Could you check a few things on this model? Use its own coordinates, in mm. A direction names the side the tool comes from. Give positions to 0.01 mm unless a question says otherwise; leave off trailing zeros. Write each loop counter-clockwise with the first axis right and the second up, starting at its lowest first coordinate (ties: lowest second). Pieces come first, ordered by that corner, then holes. Notation, with made-up numbers: M 30.5,78 L 66.5,78 A21 ccw 66.5,94 Z; hole C -6.5,-29.75 d2. An arc over 180 degrees is marked long. One line per item, written item: value.
```python
from build123d import *

# Parameters (mm, degrees)
SKETCH1_W           = 74.676
SKETCH1_H           = 63.5
BOSS_EXTRUDE1_DEPTH = 27.94
SKETCH2_W           = 69.596
SKETCH2_H           = 22.86
CUT_EXTRUDE1_DEPTH  = 60.96
SKETCH3_W           = 27.94
SKETCH3_H           = 63.5
CUT_EXTRUDE2_DEPTH  = 2.54
SKETCH4_W           = 74.676
SKETCH4_H           = 12.7
CUT_EXTRUDE3_DEPTH  = 2.54
SKETCH5_W           = 2.54
SKETCH5_H           = 63.5
BOSS_EXTRUDE2_DEPTH = 12.7
SKETCH6_R           = 3.96875
CUT_EXTRUDE4_DEPTH  = 50.8


with BuildPart() as part:
    # Sketch1 → Boss-Extrude1 (new body)
    with BuildSketch(Plane.XY):
        with Locations((1.344432395, -1.20243972)):
            Rectangle(SKETCH1_W, SKETCH1_H)
    extrude(amount=BOSS_EXTRUDE1_DEPTH)

    # Sketch2 → Cut-Extrude1 (cut)
    with BuildSketch(Plane(origin=(0, 30.54756028, 0), x_dir=(1, 0, 0), z_dir=(0, 1, 0))):
        with Locations((1.344432395, -13.97)):
            Rectangle(SKETCH2_W, SKETCH2_H)
    extrude(amount=-CUT_EXTRUDE1_DEPTH, mode=Mode.SUBTRACT)

    # Sketch3 → Cut-Extrude2 (cut)
    with BuildSketch(Plane.XY.offset(27.94)):
        with Locations((1.344432395, -1.20243972)):
            Rectangle(SKETCH3_W, SKETCH3_H)
    extrude(amount=-CUT_EXTRUDE2_DEPTH, mode=Mode.SUBTRACT)

    # Sketch4 → Cut-Extrude3 (cut)
    with BuildSketch(Plane(origin=(0, 0, 0), x_dir=(-1, 0, 0), z_dir=(0, 0, -1))):
        with Locations((-1.344432395, -26.60243972)):
            Rectangle(SKETCH4_W, SKETCH4_H)
    extrude(amount=-CUT_EXTRUDE3_DEPTH, mode=Mode.SUBTRACT)

    # Sketch5 → Boss-Extrude2 (add)
    with BuildSketch(Plane.XY.offset(27.94)):
        with Locations((-13.895567605, -1.20243972)):
            Rectangle(SKETCH5_W, SKETCH5_H)
        with Locations((16.584432395, -1.20243972)):
            Rectangle(SKETCH5_W, SKETCH5_H)
    extrude(amount=BOSS_EXTRUDE2_DEPTH)

    # Sketch6 → Cut-Extrude4 (cut)
    with BuildSketch(Plane.ZY.offset(15.165567605)):
        with Locations(Location((34.29, 17.84756028, 0), (0, 0, 270))):
            Circle(SKETCH6_R)
        with Locations(Location((34.29, -20.25243972, 0), (0, 0, 270))):
            Circle(SKETCH6_R)
    extrude(amount=-CUT_EXTRUDE4_DEPTH, mode=Mode.SUBTRACT)


solid = part.part
```
1) On a 3-axis mill with a long thin cutter (end or side, diameter ignored), from which of +Z, -Z, +X, -X, +Y, -Y can I reach the whole of each face in a straight line? I mean faces 5 (the face through (2, -20.252, 1)), 6 (the face through (36.142, 0, 14)), 7 (the face through (1, -32, 25.4)). Say none if no direction works.
Outcome:
face 5: -Z, +X, -X, -Y
face 6: +Y
face 7: +Z, +Y, -Y
2) We'd pull the mould along X, two halves only. Please class faces 1 (the face through (38.682, -2, 14)), 2 (the face through (15.314, -2, 33)), 3 (the face through (1, -32.952, 17)), 4 (the face through (-15.166, -2, 34)): pulls with the +X half, pulls with the -X half, needs draft (parallel to the pull), parting line crosses it, or undercut.
Outcome:
face 1: pulls with the +X half
face 2: undercut
face 3: needs draft
face 4: pulls with the -X half
3) I'm going to push flat-ended pins straight in: pin 1 (2 mm diameter, centred on x = 4.5, y = -31.5, fed in from +Z); pin 2 (1 mm diameter, centred on x = -18.5, y = 16.5, fed in from +Z); pin 3 (14 mm diameter, centred on y = -15, z = 35, fed in from +X); pin 4 (8 mm diameter, centred on x = 24, z = 34.5, fed in from -Y). Where does each tip first touch, or does it pass through?
Outcome:
pin 1: stops at z = 25.4
pin 2: stops at z = 27.94
pin 3: stops at x = 17.85
pin 4: passes through
4) If we section it at A-A, the plane y = -25.5: Write out the boundary of the cut face in (x, z).
Outcome:
outline: M -35.99,2.54 L -33.45,2.54 L -33.45,25.4 L -12.63,25.4 L -12.63,40.64 L -15.17,40.64 L -15.17,27.94 L -35.99,27.94 Z; M 15.31,25.4 L 36.14,25.4 L 36.14,2.54 L 38.68,2.54 L 38.68,27.94 L 17.85,27.94 L 17.85,40.64 L 15.31,40.64 Z
5) Please list where these lines run through material, in increasing order: L1, parallel to Z at x = 31, y = 24; L2, parallel to X at y = -9.5, z = 32.5; L3, parallel to Y at x = 16, z = 34. Write a range as from..to.
Outcome:
L1: z = 0..2.54, 25.4..27.94
L2: x = -15.17..-12.63, 15.31..17.85
L3: y = -32.95..-24.21, -16.29..13.89, 21.81..30.55
6) If we section it at B-B, the plane z = 34.29: Write out the boundary of the cut face in (x, y), then the cut area to 3 significant figures.
Outcome:
outline: M -15.17,-32.95 L -12.63,-32.95 L -12.63,-24.22 L -15.17,-24.22 Z; M -15.17,-16.28 L -12.63,-16.28 L -12.63,13.88 L -15.17,13.88 Z; M -15.17,21.82 L -12.63,21.82 L -12.63,30.55 L -15.17,30.55 Z; M 15.31,-32.95 L 17.85,-32.95 L 17.85,-24.22 L 15.31,-24.22 Z; M 15.31,-16.28 L 17.85,-16.28 L 17.85,13.88 L 15.31,13.88 Z; M 15.31,21.82 L 17.85,21.82 L 17.85,30.55 L 15.31,30.55 Z
area: 242 mm^2
7) If we section it at D-D, the plane z = 9.5: Write out the boundary of the cut face in (x, y).
Outcome:
outline: M -35.99,-32.95 L 38.68,-32.95 L 38.68,30.55 L 36.14,30.55 L 36.14,-30.41 L -33.45,-30.41 L -33.45,30.55 L -35.99,30.55 Z
8) If we section it at C-C, the plane x = 1.5: Write out the boundary of the cut face in (y, z), then the cut area to 3 significant figures.
Outcome:
outline: M -32.95,2.54 L -30.41,2.54 L -30.41,25.4 L -32.95,25.4 Z; M -20.25,0 L 30.55,0 L 30.55,2.54 L -20.25,2.54 Z
area: 187 mm^2
